Read the model definition and answer for the solid it produces. Units are mm, in the model's axes. A direction names the side the tool comes from. Coordinates: 2 decimals unless noted, no trailing zeros. Order: outer loops, then holes, each group sorted by start corner. A loop starts at its lowest first (then second) coordinate and runs counter-clockwise, first axis right, second up. Notation, with made-up numbers: (30, 80) -> (65, 80) arc R25 cw to (65, 113) -> close; hole circle Ø4 at (-31.75, -37). An arc over 180 degrees is marked (long way). Use CSV: the item, a comma, the result in double quotes.
Autodesk Inventor part; units mm, degrees
ref_plane "Work Plane1" through (0, 0, 0) normal (0, 1, 0) x (-1, 0, 0)
ref_plane "YZ Plane" through (0, 0, 0) normal (1, 0, 0) x (0, 1, 0)
ref_plane "XY Plane" through (0, 0, 0) normal (0, 0, 1) x (1, 0, 0)
sketch "Sketch1" plane through (0, 0, 0) normal (1, 0, 0) x (0, 1, 0)
  circle A0 centre (0, 0) radius 3.75
  dimension "d0" = 7.5
extrude "Extrusion1" add sketch "Sketch1" along normal blind 40
sketch "Sketch2" plane through (40, 0, 0) normal (1, 0, 0) x (0, 0, -1)
  circle A0 centre (0, 0) radius 3
  dimension "d3" = 6
extrude "Extrusion2" add sketch "Sketch2" along normal blind 10
chamfer "Chamfer1" distance 1.25 angle 45 1 edges at (50, 0, 3)
ref_plane "Work Plane1" through (0, 0, 0) normal (0, 1, 0) x (-1, 0, 0)
sketch "Sketch3" plane through (0, 0, 0) normal (0, 1, 0) x (-1, 0, 0)
  circle A0 centre (-45.3317, 0) radius 2
  point P0 (0, 0)
  dimension "d10" = 4
extrude "Extrusion3" cut sketch "Sketch3" along normal mid plane 10
properties part number "2nd extender"
Item 1: A tool of negligible diameter and unlimited length cuts with its end or side. For faces 4 (the cylindrical face through (44.3, 1.8, 2.4)), 5 (the cylindrical face through (19.72, -3.746, -0.165)), from which of +Z, -Z, +X, -X, +Y, -Y can it reach the whole face along a straight path? Write none if from no direction.
Return value:
face 4,"+X"
face 5,"+X, -X"
Item 2: This flat-tipped pin is pushed along its axis until it touches: P1, Ø1.5, axis at x = 17, y = 1.5, coming from the +Z side. Where does it stop, or does it pass through?
Return value:
P1,"stops at z = 3.67"
Item 3: Find section A-A, the plane z = 0. Give the vertices of the cut face in (x, y).
Return value:
outline,"(0, -3.75) -> (40, -3.75) -> (40, -3) -> (43.33, -3) -> (43.33, 3) -> (40, 3) -> (40, 3.75) -> (0, 3.75) -> close; (47.33, -3) -> (48.75, -3) -> (50, -1.75) -> (50, 1.75) -> (48.75, 3) -> (47.33, 3) -> close"
Item 4: Straight lines are drawn through the part: line 1 along X through (y, z) = (1, 0); line 2 along X through (y, z) = (-1, -0.5); line 3 along X through (y, z) = (2, 2.75). For each, find the intervals that lie inside material, in ascending order.
Return value:
line 1,"x = 0 to 43.33, 47.33 to 50"
line 2,"x = 0 to 43.4, 47.27 to 50"
line 3,"x = 0 to 40"
Item 5: Find section D-D, the plane x = 15. Give the vertices of the cut face in (y, z), then the cut area to 3 significant figures.
Return value:
outline,"circle Ø7.5 at (0, 0)"
area,"44.2 mm^2"
Item 6: Find section B-B, the plane y = 0. Give the vertices of the cut face in (x, z), then the cut area to 3 significant figures.
Return value:
outline,"(0, -3.75) -> (40, -3.75) -> (40, -3) -> (48.75, -3) -> (50, -1.75) -> (50, 1.75) -> (48.75, 3) -> (40, 3) -> (40, 3.75) -> (0, 3.75) -> close; hole circle Ø4 at (45.33, 0)"
area,"346 mm^2"
Item 7: The mould has two halves that part along X. Classify faces 1 (the cylindrical face through (46.919, 0.042, -1.217)), 2 (the flat face through (50, 0, 0)), 3 (the flat face through (0, 0, 0)): +X half, -X half, draft (parallel to the pull), parting line (faces both ways), or undercut.
Return value:
face 1,"undercut"
face 2,"+X half"
face 3,"-X half"
Item 8: Find section C-C, the plane x = 44.5. Give the vertices of the cut face in (y, z).
Return value:
outline,"(-2.39, -1.82) arc R3 ccw to (2.39, -1.82) -> close; (-2.39, 1.82) -> (2.39, 1.82) arc R3 ccw to start"
